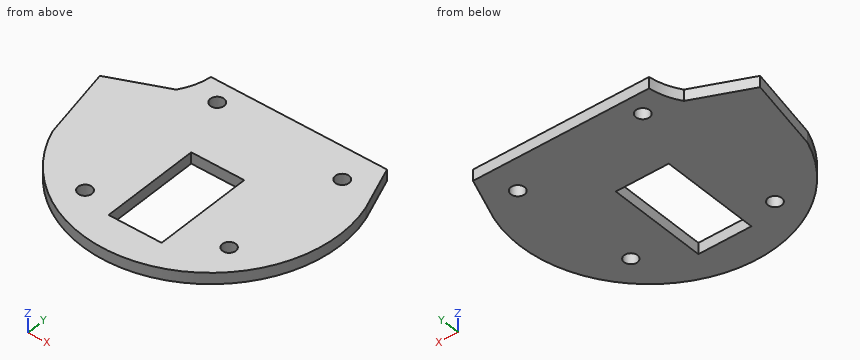
from build123d import *

# Parameters (mm, degrees)
SKETCH5_R      = 1.397
SKETCH5_R_2    = 1.362219034
EXTRUDE1_DEPTH = 2.286
SKETCH10_W     = 10.7696
SKETCH10_H     = 20.1676
EXTRUDE2_DEPTH = 2.286


with BuildPart() as part:
    # Sketch5 → Extrude1 (new body)
    with BuildSketch(Plane(origin=(0, 0, 0), x_dir=(-0.018375543, 0.999831155, 0), z_dir=(0, 0, -1))):
        with BuildLine():
            Line((33.80665155, 26.18621859), (34.46394605, -9.577814671))
            ThreePointArc((34.46394605, -9.577814671), (31.404055355, -10.348947358), (28.630167887, -11.853315998))
            Line((28.630167887, -11.853315998), (23.830153765, -23.292701447))
            Line((23.830153765, -23.292701447), (8.486225874, -20.477486777))
            ThreePointArc((8.486225874, -20.477486777), (-7.865336256, 12.262044577), (24.425706506, 29.482353943))
            Line((24.425706506, 29.482353943), (33.80665155, 26.18621859))
        make_face()
        with Locations((27.527734531, 22.260177192)):
            Circle(SKETCH5_R, mode=Mode.SUBTRACT)
        with Locations((30.179746314, -4.890797216)):
            Circle(SKETCH5_R, mode=Mode.SUBTRACT)
        with Locations((3.363138785, 18.996048152)):
            Circle(SKETCH5_R_2, mode=Mode.SUBTRACT)
        with Locations((0.317842079, -7.407837933)):
            Circle(SKETCH5_R, mode=Mode.SUBTRACT)
    extrude(amount=EXTRUDE1_DEPTH)

    # Sketch10 → Extrude2 (cut)
    with BuildSketch(Plane(origin=(0, 0, -2.286), x_dir=(-1, 0, 0), z_dir=(0, 0, -1))):
        with Locations((-4.719875056, 7.916929458)):
            Rectangle(SKETCH10_W, SKETCH10_H)
    extrude(amount=-EXTRUDE2_DEPTH, mode=Mode.SUBTRACT)


solid = part.part
Geometry check sheet. Reference: the model listing, model coordinates, mm. Coordinates: 2 decimals unless noted, no trailing zeros. Order: outer loops, then holes, each group sorted by start corner. A loop starts at its lowest first (then second) coordinate and runs counter-clockwise, first axis right, second up. Notation, with made-up numbers: (7.5, 65.25) - (66.5, 65.25) arc R15 ccw to (66.5, 82.25) - close; hole circle Ø11 at (56.25, 78). An arc over 180 degrees is marked (long way). One line per item, written item: value.
(1) Sectioned sample at D-D (x = -15). Enter the section's corners in (y, z), and give its area (3 significant figures).
Data:
outline: (-0.91, -2.29) - (27.25, -2.29) - (27.25, 0) - (-0.91, 0) - close
area: 64.4 mm^2
(2) Depth check by flat-ended pin: pin 1 Ø0.7 at (x, z) = (5.5, -0.5) entering from -Y. Enter the tip coordinate at first touch or a pass-through.
Data:
pin 1: stops at y = -9
(3) Sectioned sample at C-C (z = -1.45). Enter the section's corners in (x, y).
Data:
outline: (-23.73, 23.4) - (-20.63, 8.11) arc R26.23 ccw to (29.03, 24.96) - (25.56, 34.28) - (-10.21, 34.28) arc R12.65 cw to (-12.38, 28.41) - close; hole circle Ø2.79 at (-7.41, 0.18); hole circle Ø2.79 at (-5.44, 30.08); hole (-0.66, -2.17) - (10.1, -2.17) - (10.1, 18) - (-0.66, 18) - close; hole circle Ø2.72 at (18.93, 3.71); hole circle Ø2.79 at (21.75, 27.93)
(4) Sectioned sample at B-B (y = 9.5). Enter the section's corners in (x, z).
Data:
outline: (-20.91, -2.29) - (-0.66, -2.29) - (-0.66, 0) - (-20.91, 0) - close; (10.1, -2.29) - (29.05, -2.29) - (29.05, 0) - (10.1, 0) - close
(5) Thickness scan on probe 1 along X at (y, z) = (4.5, -0.85); probe 2 along X at (y, z) = (3, -1.85); probe 3 along X at (y, z) = (30.5, -0.1). Record the ranges inside material, lowest first. Write a range as from..to.
Data:
probe 1: x = -18.98..-0.66, 10.1..17.82, 20.04..26.92
probe 2: x = -18.08..-0.66, 10.1..17.77, 20.09..26.03
probe 3: x = -11.21..-6.78, -4.11..26.97
(6) Sectioned sample at A-A (x = 5). Enter the section's corners in (y, z).
Data:
outline: (-9.01, -2.29) - (-2.17, -2.29) - (-2.17, 0) - (-9.01, 0) - close; (18, -2.29) - (34.28, -2.29) - (34.28, 0) - (18, 0) - close
